Autodesk Inventor part; units mm, degrees
ref_plane "YZ Plane" through (0, 0, 0) normal (1, 0, 0) x (0, 1, 0)
ref_plane "XZ Plane" through (0, 0, 0) normal (0, 1, 0) x (-1, 0, 0)
ref_plane "XY Plane" through (0, 0, 0) normal (0, 0, 1) x (1, 0, 0)
sketch "Sketch1" plane through (0, 0, 0) normal (0, 1, 0) x (-1, 0, 0)
  circle A0 centre (0, 0) radius 2
  dimension "d0" = 4
extrude "Extrusion1" add sketch "Sketch1" along normal blind 12.5
sketch "Sketch2" plane through (0, 12.5, 0) normal (0, 1, 0) x (1, 0, 0)
  circle A0 centre (0, 0) radius 3
  dimension "d3" = 6
extrude "Extrusion2" add sketch "Sketch2" along normal blind 5
sketch "Sketch3" plane through (0, 17.5, 0) normal (0, 1, 0) x (1, 0, 0)
  circle A0 centre (0, 0) radius 2
  line L0 (0, 2) -> (1.7321, 1)
  line L1 (1.7321, 1) -> (1.7321, -1)
  line L2 (1.7321, -1) -> (0, -2)
  line L3 (0, -2) -> (-1.7321, -1)
  line L4 (-1.7321, -1) -> (-1.7321, 1)
  line L5 (-1.7321, 1) -> (0, 2)
extrude "Extrusion3" cut sketch "Sketch3" against normal blind 1.5 contours L1 L2 L3 L4 L5 L0
thread "Thread1"
properties part number "4mm_0.5_Screw"
The listing builds one solid part. Answer for the finished solid, in the listing's coordinates (mm). A direction names the side the tool comes from. Round coordinates to 2 decimals unless told otherwise and drop trailing zeros. Order: outer loops, then holes, each group sorted by start corner. A loop starts at its lowest first (then second) coordinate and runs counter-clockwise, first axis right, second up. Notation, with made-up numbers: (-3.75, 7) - (19.25, 7) arc R15 cw to (19.25, 35) - close; hole circle Ø4 at (-31, -9.75). An arc over 180 degrees is marked (long way). Put each result on its own line as item: value. Start each with the question number.
(1) Find section D-D (y = 14.75). Give the vertices of the cut face in (x, z).
(2) For faces 1 (the cylindrical face through (-3, 15, 0)), 2 (the flat face through (1, 12.5, 2)), 3 (the flat face through (0.88, 16.76, 1.49)), determine the directions among +Z, -Z, +X, -X, +Y, -Y from which every point of the face is accessible in a straight line to the end or side of a thin tool.
(3) Straight lines are drawn through the part: probe 1 along Y at (x, z) = (0.45, -0.2); probe 2 along Y at (x, z) = (-2, -0.7); probe 3 along X at (y, z) = (6, -0.1). For each, find the intervals that lie inside material, in ascending order. Write a range as from..to.
(4) Determine the mould class of faces 4 (the cylindrical face through (0, 6, 2)), 5 (the flat face through (-0.85, 16.76, 1.51)), 6 (the flat face through (0, 0, 0)) for opening direction Z: released by +Z, released by -Z, zero draft, split by the parting line, or undercut.
(5) Find section A-A (z = 0). Give the vertices of the cut face in (x, y), plus the area to 3 significant figures.
(6) Find section B-B (x = -0.9). Give the vertices of the cut face in (y, z), plus the area to 3 significant figures.
(7) Find section C-C (y = 9). Give the vertices of the cut face in (x, z), plus the area to 3 significant figures.
(8) Given P1, Ø1, axis at x = -0.5, z = -1, coming from the +Y side; P2, Ø3, axis at y = 10, z = 1.5, coming from the +X side; P3, Ø2, axis at x = -2, y = 14.5, coming from the +Z side, each flat-ended and moving along its own axis, determine where each tip first touches the part or whether it passes through.
Reply:
1. outline: circle Ø6 at (0, 0)
2. face 1: +Y, -Y
2. face 2: -Y
2. face 3: +Y
3. probe 1: 0..16
3. probe 2: 12.5..17.5
3. probe 3: -2..2
4. face 4: split by the parting line
4. face 5: undercut
4. face 6: zero draft
5. outline: (-3, 12.5) - (-2, 12.5) - (-2, 0) - (2, 0) - (2, 12.5) - (3, 12.5) - (3, 17.5) - (1.73, 17.5) - (1.73, 16) - (-1.73, 16) - (-1.73, 17.5) - (-3, 17.5) - close
5. area: 74.8 mm^2
6. outline: (0, -1.79) - (12.5, -1.79) - (12.5, -2.86) - (17.5, -2.86) - (17.5, -1.48) - (16, -1.48) - (16, 1.48) - (17.5, 1.48) - (17.5, 2.86) - (12.5, 2.86) - (12.5, 1.79) - (0, 1.79) - close
6. area: 68.8 mm^2
7. outline: circle Ø4 at (0, 0)
7. area: 12.6 mm^2
8. P1: y = 16
8. P2: x = 2
8. P3: z = 2.83
